```python
from build123d import *

# Parameters (mm, degrees)
BOSS_EXTRUDE1_DEPTH     = 3.175
CUT_EXTRUDE1_DEPTH      = 339.893140422
CUT_EXTRUDE1_DEPTH_BACK = 339.893140422
SKETCH3_R               = 2.38125


with BuildPart() as part:
    # Sketch2 → Boss-Extrude1 (new body)
    with BuildSketch(Plane(origin=(0, 0, 0), x_dir=(1, 0, 0), z_dir=(0, 1, 0))):
        Polygon((22.0265625, 25.4), (72.8265625, 76.2), (123.6265625, 76.2), (174.4265625, 25.4), (330.2, 25.4), (330.2, -25.4), (174.4265625, -25.4), (123.6265625, -76.2), (72.8265625, -76.2), (22.0265625, -25.4), (-22.0265625, -25.4), (-72.8265625, -76.2), (-123.6265625, -76.2), (-174.4265625, -25.4), (-330.2, -25.4), (-330.2, 25.4), (-174.4265625, 25.4), (-123.6265625, 76.2), (-72.8265625, 76.2), (-22.0265625, 25.4), align=None)
    extrude(amount=BOSS_EXTRUDE1_DEPTH)

    # Sketch3 → Cut-Extrude1 (cut, two sides: drawn at the far end of the back side and taken through both)
    with BuildSketch(Plane(origin=(0, 3.175, 0), x_dir=(1, 0, 0), z_dir=(0, 1, 0)).offset(-CUT_EXTRUDE1_DEPTH_BACK)):
        with Locations(Location((-110.9265625, 63.5, 0), (0, 0, 270))):
            Circle(SKETCH3_R)
        with Locations(Location((-85.5265625, 63.5, 0), (0, 0, 270))):
            Circle(SKETCH3_R)
        with Locations(Location((-110.9265625, 38.1, 0), (0, 0, 270))):
            Circle(SKETCH3_R)
        with Locations(Location((-85.5265625, 38.1, 0), (0, 0, 270))):
            Circle(SKETCH3_R)
        with Locations(Location((-85.5265625, -38.1, 0), (0, 0, 270))):
            Circle(SKETCH3_R)
        with Locations(Location((-110.9265625, -38.1, 0), (0, 0, 270))):
            Circle(SKETCH3_R)
        with Locations(Location((-85.5265625, -63.5, 0), (0, 0, 270))):
            Circle(SKETCH3_R)
        with Locations(Location((-110.9265625, -63.5, 0), (0, 0, 270))):
            Circle(SKETCH3_R)
        with Locations(Location((110.9265625, -63.5, 0), (0, 0, 270))):
            Circle(SKETCH3_R)
        with Locations(Location((85.5265625, -63.5, 0), (0, 0, 270))):
            Circle(SKETCH3_R)
        with Locations(Location((110.9265625, -38.1, 0), (0, 0, 270))):
            Circle(SKETCH3_R)
        with Locations(Location((85.5265625, -38.1, 0), (0, 0, 270))):
            Circle(SKETCH3_R)
        with Locations(Location((85.5265625, 38.1, 0), (0, 0, 270))):
            Circle(SKETCH3_R)
        with Locations(Location((110.9265625, 38.1, 0), (0, 0, 270))):
            Circle(SKETCH3_R)
        with Locations(Location((85.5265625, 63.5, 0), (0, 0, 270))):
            Circle(SKETCH3_R)
        with Locations(Location((110.9265625, 63.5, 0), (0, 0, 270))):
            Circle(SKETCH3_R)
        with Locations(Location((-292.1, -12.7, 0), (0, 0, 270))):
            Circle(SKETCH3_R)
        with Locations(Location((-317.5, -12.7, 0), (0, 0, 270))):
            Circle(SKETCH3_R)
        with Locations(Location((-317.5, 12.7, 0), (0, 0, 270))):
            Circle(SKETCH3_R)
        with Locations(Location((-292.1, 12.7, 0), (0, 0, 270))):
            Circle(SKETCH3_R)
        with Locations(Location((292.1, 12.7, 0), (0, 0, 270))):
            Circle(SKETCH3_R)
        with Locations(Location((317.5, 12.7, 0), (0, 0, 270))):
            Circle(SKETCH3_R)
        with Locations(Location((317.5, -12.7, 0), (0, 0, 270))):
            Circle(SKETCH3_R)
        with Locations(Location((292.1, -12.7, 0), (0, 0, 270))):
            Circle(SKETCH3_R)
        with Locations(Location((-12.7, 12.7, 0), (0, 0, 270))):
            Circle(SKETCH3_R)
        with Locations(Location((12.7, 12.7, 0), (0, 0, 270))):
            Circle(SKETCH3_R)
        with Locations(Location((12.7, -12.7, 0), (0, 0, 270))):
            Circle(SKETCH3_R)
        with Locations(Location((-12.7, -12.7, 0), (0, 0, 270))):
            Circle(SKETCH3_R)
    extrude(amount=CUT_EXTRUDE1_DEPTH + CUT_EXTRUDE1_DEPTH_BACK, mode=Mode.SUBTRACT)


solid = part.part
```
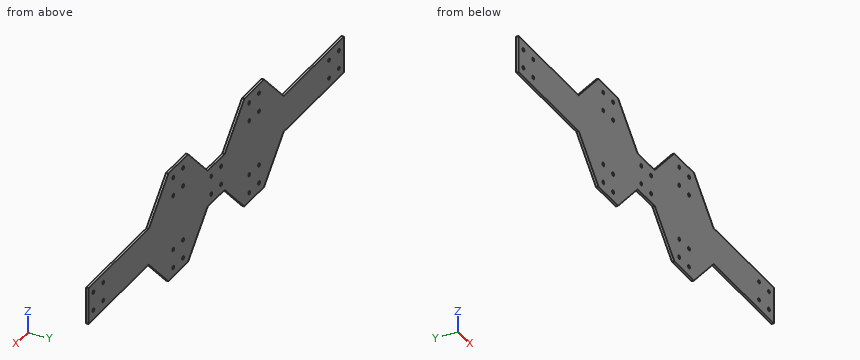
Here's how the part is built. I have some questions about the finished solid (model axes, mm). Give positions to 0.01 mm unless a question says otherwise; leave off trailing zeros. Order: outer loops, then holes, each group sorted by start corner. A loop starts at its lowest first (then second) coordinate and runs counter-clockwise, first axis right, second up. Notation, with made-up numbers: (17.5, 60) -> (41.5, 60) arc R28 ccw to (41.5, 87) -> close; hole circle Ø8 at (14.5, -22.5). An arc over 180 degrees is marked (long way). Use CSV: the item, a comma, the result in double quotes. Start each with the question number.
Item 1: If I drill on probe 1 along Z at (x, y) = (-292.1, 2); probe 2 along X at (y, z) = (2.5, 38.1); probe 3 along X at (y, z) = (1.5, 63.5), over which ranges is the centre line in solid material (lowest first)? Write a range as [from, to].
Item 2: Suppose I cut it at A-A (z = -46). List the corners of the cut face in (x, y) for me (3 decimals).
Item 3: Suppose I cut it at D-D (x = 57). List the corners of the cut face in (y, z) for me (3 decimals).
Item 4: Suppose I cut it at C-C (y = 0.8). Give the number of separate pieces and of enclosed holes in the cut face, and give its area (3 significant figures).
Item 5: I'm going to push flat-ended pins straight in: P1, Ø3, axis at x = -85.53, z = -38.1, coming from the +Y side; P2, Ø1.5, axis at x = -253, y = 2.5, coming from the +Z side. Where does each tip first touch, or does it pass through?
Item 6: Suppose I cut it at B-B (x = 265). List the corners of the cut face in (y, z) for me (3 decimals), and give its area (3 significant figures).
Answer block:
1,probe 1,"z = [-25.4, -15.08], [-10.32, 10.32], [15.08, 25.4]"
1,probe 2,"x = [-161.73, -113.31], [-108.55, -87.91], [-83.15, -34.73], [34.73, 83.15], [87.91, 108.55], [113.31, 161.73]"
1,probe 3,"x = [-136.33, -113.31], [-108.55, -87.91], [-83.15, -60.13], [60.13, 83.15], [87.91, 108.55], [113.31, 136.33]"
2,outline,"(-153.827, 0) -> (-42.627, 0) -> (-42.627, 3.175) -> (-153.827, 3.175) -> close; (42.627, 0) -> (153.827, 0) -> (153.827, 3.175) -> (42.627, 3.175) -> close"
3,outline,"(0, -60.373) -> (3.175, -60.373) -> (3.175, 60.373) -> (0, 60.373) -> close"
4,separate pieces,"1"
4,enclosed holes,"28"
4,area,"53,700 mm^2"
5,P1,"passes through"
5,P2,"stops at z = 25.4"
6,outline,"(0, -25.4) -> (3.175, -25.4) -> (3.175, 25.4) -> (0, 25.4) -> close"
6,area,"161 mm^2"
